Read the model definition and answer for the solid it produces. Units are mm, in the model's axes. Face numbers are marked on the shaded views. A direction names the side the tool comes from. Round coordinates to 2 decimals unless told otherwise and drop trailing zeros. Order: outer loops, then holes, each group sorted by start corner. A loop starts at its lowest first (then second) coordinate and runs counter-clockwise, first axis right, second up. Notation, with made-up numbers: (57.25, -23) - (106.25, -23) arc R12 ccw to (106.25, -7) - close; hole circle Ø10 at (65, 23). An arc over 180 degrees is marked (long way). Put each result on its own line as item: value. Start each with the question number.
Q1. Each of these flat-tipped pins is pushed along its axis until it touches: pin 1 Ø5 at (y, z) = (93.5, -6) entering from -X; pin 2 Ø12 at (x, z) = (23, -10) entering from +Y; pin 3 Ø7.5 at (y, z) = (10.5, -11) entering from +X. Where does it stop, or does it pass through?
Q2. Section A-A on x = 26.5 is taken. Give the vertices of the cut face in (y, z).
Q3. Find the intervals of material crossed by line 1 along Z through (x, y) = (19, 15.5); line 2 along Y through (x, z) = (48, -17.25); line 3 along Z through (x, y) = (45, 128), in increasing order. Write a range as from..to.
Q4. Section C-C on x = 38 is taken. Give the vertices of the cut face in (y, z), then the cut area to 3 significant figures.
Q5. Which of the six approach directions +Z, -Z, +X, -X, +Y, -Y give full straight-line access (tool end or side, diameter ignored) to the marked faces 1, 2, 3, 4 and 5?
Q6. Section B-B on y = 37 is taken. Give the vertices of the cut face in (x, z).
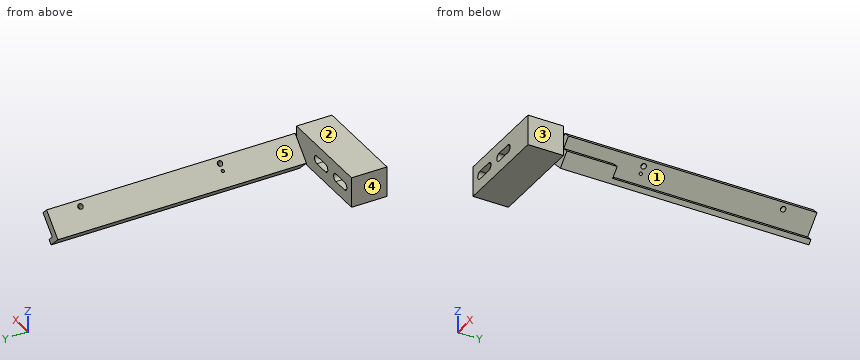
from build123d import *

# Parameters (mm, degrees)
SKETCH1_W                             = 48.26
SKETCH1_H                             = 17.78
BOSS_EXTRUDE1_DEPTH                   = 15.24
CUT_EXTRUDE2_DEPTH                    = 54.641528688
BOSS_EXTRUDE2_DEPTH                   = 124.7199944
BOSS_EXTRUDE4_DEPTH                   = 18.21999912
BOSS_EXTRUDE5_DEPTH                   = 25.2199902
F_1_5MM_DOWEL_HOLE1_D                 = 1.5
TAPPED_HOLE_FOR_M2_5X0_45_HELICOIL1_D = 2.55


with BuildPart() as part:
    # Sketch1 → Boss-Extrude1 (new body)
    with BuildSketch(Plane.XY):
        with Locations((24.13, 8.89)):
            Rectangle(SKETCH1_W, SKETCH1_H)
    extrude(amount=-BOSS_EXTRUDE1_DEPTH)

    # Sketch4 → Cut-Extrude2 (cut, through all)
    with BuildSketch(Plane(origin=(0, 17.78, 0), x_dir=(1, 0, 0), z_dir=(0, 1, 0))):
        with BuildLine():
            Line((30.48, 5.62), (22.86, 5.62))
            ThreePointArc((22.86, 5.62), (20.86, 7.62), (22.86, 9.62))
            Line((22.86, 9.62), (30.48, 9.62))
            ThreePointArc((30.48, 9.62), (32.48, 7.62), (30.48, 5.62))
        make_face()
        with BuildLine():
            Line((13.78, 5.62), (6.16, 5.62))
            ThreePointArc((6.16, 5.62), (4.16, 7.62), (6.16, 9.62))
            Line((6.16, 9.62), (13.78, 9.62))
            ThreePointArc((13.78, 9.62), (15.78, 7.62), (13.78, 5.62))
        make_face()
    extrude(amount=-CUT_EXTRUDE2_DEPTH, mode=Mode.SUBTRACT)

    # Sketch3 → Boss-Extrude2 (add)
    with BuildSketch(Plane(origin=(0, 17.78, 0), x_dir=(1, 0, 0), z_dir=(0, 1, 0))):
        Polygon((52.660828417, 7.619998743), (48.488883403, 11.791943757), (44.529097479, 15.751729681), (47.357520181, 18.580152383), (45.561468957, 20.376203607), (40.42526535, 15.24), (39.573657012, 14.388391662), (49.501439174, 4.4606095), align=None)
    extrude(amount=BOSS_EXTRUDE2_DEPTH)

    # Sketch3<7> → Boss-Extrude4 (add)
    with BuildSketch(Plane(origin=(0, 17.78, 0), x_dir=(1, 0, 0), z_dir=(0, 1, 0))):
        Polygon((39.573657012, 14.388391662), (40.42526535, 15.24), (45.561468957, 20.376203607), (47.357520181, 18.580152383), (44.529097479, 15.751729681), (52.660828417, 7.619998743), (49.501439174, 4.4606095), align=None)
    extrude(amount=BOSS_EXTRUDE4_DEPTH)

    # Sketch3<8> → Boss-Extrude5 (add)
    with BuildSketch(Plane(origin=(0, 17.78, 0), x_dir=(1, 0, 0), z_dir=(0, 1, 0))):
        Polygon((44.529097479, 15.751729681), (48.488883403, 11.791943757), (51.317306105, 14.620366459), (47.357520181, 18.580152383), align=None)
    extrude(amount=BOSS_EXTRUDE5_DEPTH)

    # Ø1.5mm Dowel Hole1 (through all)
    with Locations(Plane(origin=(30.14041358, 0, -30.14041358), x_dir=(-0.707106781186544, 0, -0.7071067811865511), z_dir=(0.7071067811865511, 0, -0.707106781186544))):
        with Locations((-25.348661915, 56.6999882)):
            Hole(F_1_5MM_DOWEL_HOLE1_D / 2)

    # Tapped Hole for M2.5x0.45 Helicoil1 (through all)
    with Locations(Plane(origin=(30.14041358, 0, -30.14041358), x_dir=(-0.7071067811865478, 0, -0.7071067811865472), z_dir=(0.7071067811865472, 0, -0.7071067811865478))):
        with Locations((-28.898667515, 56.6999882), (-28.898667515, 126.6998482)):
            Hole(TAPPED_HOLE_FOR_M2_5X0_45_HELICOIL1_D / 2)


solid = part.part
Findings:
1. pin 1: x = 45.46
1. pin 2: y = 17.78
1. pin 3: x = 48.26
2. outline: (0, -15.24) - (17.78, -15.24) - (17.78, -9.62) - (0, -9.62) - close; (0, -5.62) - (17.78, -5.62) - (17.78, 0) - (0, 0) - close
3. line 1: -15.24..0
3. line 2: 17.78..43
3. line 3: -19.81..-16.22, -15.28..-8.96
4. outline: (0, -15.24) - (17.78, -15.24) - (17.78, 0) - (0, 0) - close
4. area: 271 mm2
5. face 1: +X, +Y
5. face 2: +Z, +X, -X, +Y, -Y
5. face 3: +Z, -Z, +X, -Y
5. face 4: +Z, -Z, -X, +Y, -Y
5. face 5: +Z, -X, +Y
6. outline: (39.57, -14.39) - (45.56, -20.38) - (51.32, -14.62) - (48.49, -11.79) - (52.66, -7.62) - (49.5, -4.46) - close
